from build123d import *

# Parameters (mm, degrees)
F1_DEPTH = 4


with BuildPart() as f1:
    # F0 (on Front) → F1 (new body)
    with BuildSketch(Plane.XZ):
        Polygon((18.1212967897, 0), (19.5590760559, 0), (18.8588984311, 1.6234545037), align=None)
        with BuildLine():
            Line((19.5590760559, -2.1580299363), (19.5590760559, 0))
            Line((19.5590760559, 0), (18.1212967897, 0))
            Line((18.1212967897, 0), (16.5056623518, 0))
            Line((16.5056623518, 0), (14.9563110818, 0))
            Line((14.9563110818, 0), (13.6181200498, 0))
            Line((13.6181200498, 0), (11.6327671148, 0))
            Line((11.6327671148, 0), (-3.8659593556, 0))
            Line((-3.8659593556, 0), (-6.5012451862, 0))
            Line((-6.5012451862, 0), (-17.3736400902, 0))
            add(Edge.make_bspline(
                [(-18.5409239441, -0.7620579563), (-18.5313819873, -0.5570340705), (-18.5088219152, -0.0722955878), (-17.7890049244, -0.0264530705), (-17.3736400902, 0)],
                knots=[0, 0, 0, 0, 0.4229577248, 1, 1, 1, 1], degree=3))
            Line((-18.5409239441, -0.7620579563), (-18.5409239441, -2.4619437754))
            add(Edge.make_bspline(
                [(-18.5409239441, -2.4619437754), (-18.5568826251, -2.7188473012), (-18.5924766066, -3.2918407312), (-17.8507141613, -3.2983881425), (-17.4415233956, -3.302)],
                knots=[0, 0, 0, 0, 0.4483533532, 1, 1, 1, 1], degree=3))
            ThreePointArc((-17.4415233956, -3.302), (-14.9394255131, -2.8779800495), (-12.4373276307, -3.302))
            Line((-12.4373276307, -3.302), (18.1434545666, -3.302))
            add(Edge.make_bspline(
                [(18.1434545666, -3.302), (18.5720487525, -3.2862632294), (19.3979681291, -3.2559377976), (19.5067461789, -2.5146441916), (19.5590760559, -2.1580299363)],
                knots=[0, 0, 0, 0, 0.5189298108, 1, 1, 1, 1], degree=3))
        make_face()
        Polygon((14.9563110818, 0), (16.5056623518, 0), (15.792561695, 1.6234545037), align=None)
        Polygon((11.6327671148, 0), (13.6181200498, 0), (12.546707876, 1.6234545037), align=None)
        Polygon((-6.5012451862, 0), (-3.8659593556, 0), (-7.5336750597, 1.4574349625), (-4.2313374579, 2.2132038139), (-7.4203494005, 3.6106230691), (-3.5889614675, 4.6581615955), (-6.2896457049, 4.8301138928), (-10.1779419929, 3.7617245689), (-7.0804748294, 2.40442007), (-10.1779419929, 1.2916467484), align=None)
        with BuildLine():
            Line((-6.2896457049, 4.8301138928), (-3.5889614675, 4.6581615955))
            Line((-3.5889614675, 4.6581615955), (11.6327671148, 3.6889956474))
            Line((11.6327671148, 3.6889956474), (13.6181200498, 3.5625884231))
            Line((13.6181200498, 3.5625884231), (14.4155324855, 3.5118172525))
            Line((14.4155324855, 3.5118172525), (16.8658798656, 3.355803878))
            Line((16.8658798656, 3.355803878), (17.6075737409, 3.3085803026))
            Line((17.6075737409, 3.3085803026), (19.5355117321, 3.185828682))
            Line((19.5355117321, 3.185828682), (19.5590760559, 3.1843283439))
            Line((19.5590760559, 3.1843283439), (19.5590760559, 4.9431086518))
            add(Edge.make_bspline(
                [(18.3420831283, 6.1964309278), (18.7345885657, 6.1878547056), (19.5281427506, 6.1705155904), (19.5486912134, 5.3551702683), (19.5590760559, 4.9431086518)],
                knots=[0, 0, 0, 0, 0.4946170594, 1, 1, 1, 1], degree=3))
            Line((18.3420831283, 6.1964309278), (-12.4568440589, 8.3355969669))
            ThreePointArc((-12.4568440589, 8.3355969669), (-15.0516657643, 8.0968521777), (-17.5885669887, 8.692025207))
            add(Edge.make_bspline(
                [(-18.5409239441, 8.1570418552), (-18.5248625182, 8.314252707), (-18.4866086391, 8.6886855231), (-17.9182767751, 8.6907990651), (-17.5885669887, 8.692025207)],
                knots=[0, 0, 0, 0, 0.4198639786, 1, 1, 1, 1], degree=3))
            Line((-18.5409239441, 8.1570418552), (-18.5409239441, 6.2195211649))
            add(Edge.make_bspline(
                [(-18.5409239441, 6.2195211649), (-18.5449199509, 6.03695186), (-18.5543470455, 5.6062473591), (-17.9217358709, 5.568988424), (-17.5572792713, 5.5475230036)],
                knots=[0, 0, 0, 0, 0.4238852961, 1, 1, 1, 1], degree=3))
            Line((-17.5572792713, 5.5475230036), (-6.2896457049, 4.8301138928))
        make_face()
        Polygon((13.6181200498, 3.5625884231), (11.6327671148, 3.6889956474), (12.546707876, 1.6966089606), align=None)
        Polygon((16.8658798656, 3.355803878), (14.4155324855, 3.5118172525), (15.792561695, 1.6966089606), align=None)
        Polygon((19.5355117321, 3.185828682), (17.6075737409, 3.3085803026), (18.8588984311, 1.6966089606), align=None)
    extrude(amount=F1_DEPTH)


solid = f1.part
The listing builds one solid part. Answer for the finished solid, in the listing's coordinates (mm). A direction names the side the tool comes from. Round coordinates to 2 decimals unless told otherwise and drop trailing zeros. Write each loop counter-clockwise with the first axis right and the second up, starting at its lowest first coordinate (ties: lowest second). Pieces come first, ordered by that corner, then holes. Notation, with made-up numbers: M 31,9.5 L 71,9.5 A23 cw 71,21.5 Z; hole C 84.25,70.25 d7. An arc over 180 degrees is marked long. Write each question's results on one line, items separated by ' | '. Start each with the question number.
Item 1: Flat-ended cylindrical pins translate along their axes: pin 1 Ø1 at (x, z) = (9.5, 3) entering from +Y; pin 2 Ø0.5 at (y, z) = (-1.5, -1.5) entering from -X; pin 3 Ø0.5 at (x, y) = (17, -2.5) entering from +Z. Find the tip coordinate at first contact, or state that the pin passes through.
Item 2: Straight lines are drawn through the part: L1, parallel to Z at x = -8.5, y = -0.55; L2, parallel to X at y = -1.2, z = -0.75; L3, parallel to Z at x = 16, y = -3.05. For each, find the intervals that lie inside material, in ascending order. Write a range as [from, to].
Item 3: A cutting plane is placed at A-A on x = 2.5. Write down the section's boundary in (y, z).
Item 4: A cutting plane is placed at B-B on x = -10.5. Write down the section's boundary in (y, z).
Item 5: For a pull along Z with two mould halves and no side action, classify faces 4 (the face through (0, -4, 5)), 5 (the face through (13.09, -1.97, 0.8)), 6 (the face through (-15.015, -1.972, 8.094)) as pulls with the +Z half, pulls with the -Z half, needs draft (parallel to the pull), parting line crosses it, or undercut.
Item 6: For faces 1 (the face through (-12.002, -1.972, 5.194)), 2 (the face through (17, -2, 0)), 3 (the face through (0, 0, 5)), determine the directions among +Z, -Z, +X, -X, +Y, -Y from which every point of the face is accessible in a straight line to the end or side of a thin tool.
Check sheet entries:
1) pin 1: through | pin 2: x = -18.54 | pin 3: z = 6.31
2) L1: [-3.3, 0], [0.7, 1.89], [3.03, 4.22], [4.97, 8.06] | L2: [-18.54, 19.56] | L3: [-3.3, 1.15], [2.02, 6.36]
3) outline: M -4,-3.3 L 0,-3.3 L 0,0 L -4,0 Z; M -4,4.27 L 0,4.27 L 0,7.3 L -4,7.3 Z
4) outline: M -4,-3.3 L 0,-3.3 L 0,0 L -4,0 Z; M -4,5.1 L 0,5.1 L 0,8.2 L -4,8.2 Z
5) face 4: needs draft | face 5: undercut | face 6: pulls with the +Z half
6) face 1: -X, +Y, -Y | face 2: +Y, -Y | face 3: +Z, -Z, +X, -X, +Y
